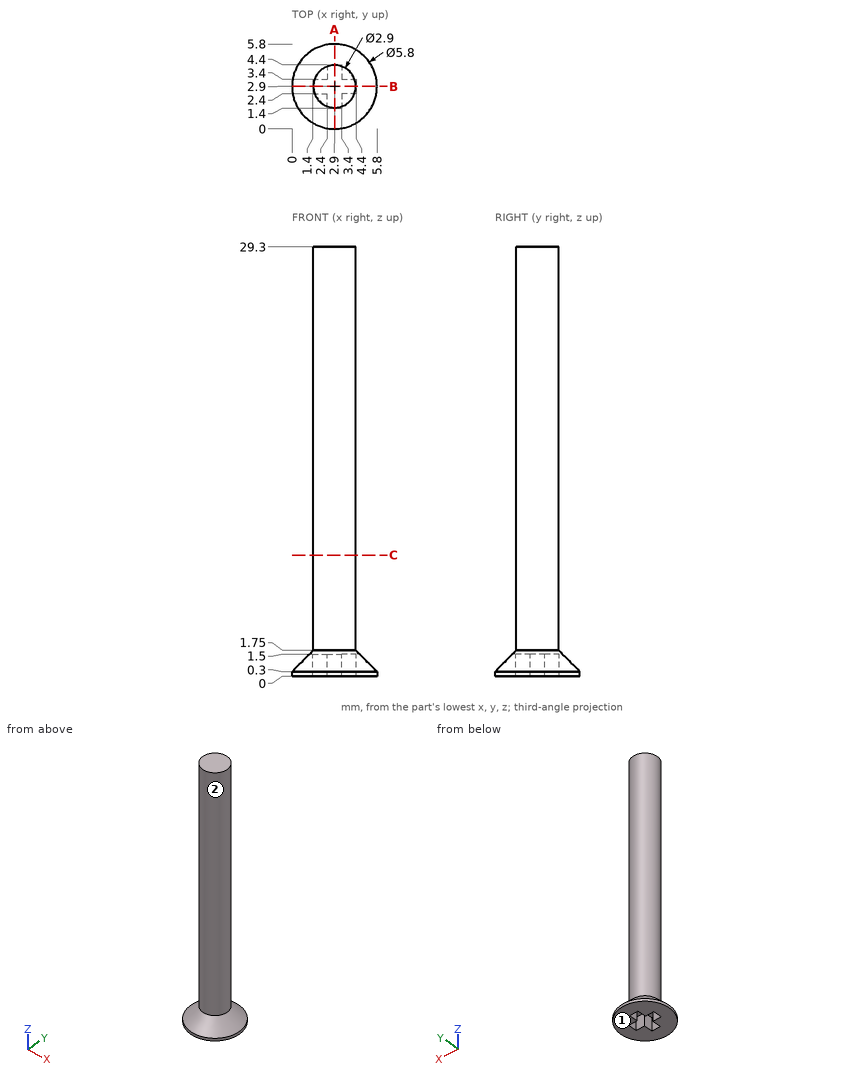
Part print with two shaded views. Sizes in mm from the minimum x, y, z corner. A direction names the side the tool comes from. Coordinates: 2 decimals unless noted, no trailing zeros. Write each loop counter-clockwise with the first axis right and the second up, starting at its lowest first coordinate (ties: lowest second). Pieces come first, ordered by that corner, then holes. Notation, with made-up numbers: (-15.5, 2) - (0.5, 2) arc R27 ccw to (0.5, 37) - close; hole circle Ø2 at (-9, -13.75). An arc over 180 degrees is marked (long way). One line per item, written item: value. Start each with the question number.
1. Tool access for the marked faces 1 and 2: list every direction of +Z, -Z, +X, -X, +Y, -Y with a clear straight run to the whole face (end or side of a thin tool).
2. Probe line 1 (Z direction, x = 3.35, y = 3.9); line 2 (Z direction, x = 0.85, y = 3.75); line 3 (X direction, y = 2.75, z = 16.5). List the from-to ranges inside material, lowest first. Write a range as from..to.
3. Flat gauge pins, fed straight in: pin 1 (1.1 mm diameter, centred on y = 3.5, z = 1, fed in from -X); pin 2 (1 mm diameter, centred on y = 4.5, z = 26, fed in from -X); pin 3 (0.8 mm diameter, centred on y = 4, z = 1, fed in from +X). Where does each tip first touch, or does it go through?
4. Slice it at A-A (x = 2.9). Write the cut outline in (y, z).
5. Slice it at C-C (z = 8.25). Write the cut outline in (x, y).
Answers below:
1. face 1: -Z, +X, -X, +Y, -Y
1. face 2: +Z
2. line 1: z = 1.5..29.3
2. line 2: z = 0..0.98
2. line 3: x = 1.46..4.34
3. pin 1: stops at x = 0.21
3. pin 2: stops at x = 1.96
3. pin 3: stops at x = 5.29
4. outline: (0, 0) - (1.4, 0) - (1.4, 1.5) - (4.4, 1.5) - (4.4, 0) - (5.8, 0) - (5.8, 0.3) - (4.35, 1.75) - (4.35, 29.3) - (1.45, 29.3) - (1.45, 1.75) - (0, 0.3) - close
5. outline: circle Ø2.9 at (2.9, 2.9)
